from build123d import *

# Parameters (mm, degrees)
SKETCH1_W           = 150
SKETCH1_H           = 45
BOSS_EXTRUDE1_DEPTH = 60
SKETCH2_W           = 70
SKETCH2_H           = 30
CUT_EXTRUDE1_DEPTH  = 60
SKETCH8_W           = 25
SKETCH8_H           = 60
CUT_EXTRUDE5_DEPTH  = 30
SKETCH9_R           = 25
BOSS_EXTRUDE4_DEPTH = 35
SKETCH10_R          = 20
SKETCH10_R_2        = 15
CUT_EXTRUDE7_DEPTH  = 10
SKETCH10_5_R        = 15
SKETCH10_5_R_2      = 10
CUT_EXTRUDE8_DEPTH  = 70
SKETCH12_R          = 5
CUT_EXTRUDE9_DEPTH  = 70
FILLET1_R           = 10
SKETCH13_R          = 7
CUT_EXTRUDE10_DEPTH = 15
SKETCH14_R          = 5
CUT_EXTRUDE11_DEPTH = 15
FILLET2_R           = 5


with BuildPart() as part:
    # Sketch1 → Boss-Extrude1 (new body)
    with BuildSketch(Plane.XY):
        Rectangle(SKETCH1_W, SKETCH1_H)
    extrude(amount=BOSS_EXTRUDE1_DEPTH)

    # Sketch2 → Cut-Extrude1 (cut)
    with BuildSketch(Plane.XY.offset(60)):
        with Locations((0, -7.5)):
            Rectangle(SKETCH2_W, SKETCH2_H)
    extrude(amount=-CUT_EXTRUDE1_DEPTH, mode=Mode.SUBTRACT)

    # Sketch8 → Cut-Extrude5 (cut)
    with BuildSketch(Plane(origin=(0, 22.5, 0), x_dir=(1, 0, 0), z_dir=(0, 1, 0))):
        with Locations((-62.5, -30)):
            Rectangle(SKETCH8_W, SKETCH8_H)
        with Locations((62.5, -30)):
            Rectangle(SKETCH8_W, SKETCH8_H)
    extrude(amount=-CUT_EXTRUDE5_DEPTH, mode=Mode.SUBTRACT)

    # Sketch9 → Boss-Extrude4 (add)
    with BuildSketch(Plane(origin=(0, 22.5, 0), x_dir=(1, 0, 0), z_dir=(0, 1, 0))):
        with Locations(Location((0, -30, 0), (0, 0, 180))):
            Circle(SKETCH9_R)
    extrude(amount=BOSS_EXTRUDE4_DEPTH)

    # Sketch10 → Cut-Extrude7 (cut)
    with BuildSketch(Plane(origin=(0, 57.5, 0), x_dir=(1, 0, 0), z_dir=(0, 1, 0))):
        with Locations(Location((0, -30, 0), (0, 0, 270))):
            Circle(SKETCH10_R)
        with Locations(Location((0, -30, 0), (0, 0, 270))):
            Circle(SKETCH10_R_2, mode=Mode.SUBTRACT)
    extrude(amount=-CUT_EXTRUDE7_DEPTH, mode=Mode.SUBTRACT)

    # Sketch10_5 → Cut-Extrude8 (cut)
    # profile 1 of 2: a face of its own
    with BuildSketch(Plane(origin=(0, 57.5, 0), x_dir=(1, 0, 0), z_dir=(0, 1, 0))):
        with Locations(Location((0, -30, 0), (0, 0, 270))):
            Circle(SKETCH10_5_R)
        with Locations((0, -30)):
            Circle(SKETCH10_5_R_2, mode=Mode.SUBTRACT)
    # profile 2 of 2: a face of its own
    with BuildSketch(Plane(origin=(0, 57.5, 0), x_dir=(1, 0, 0), z_dir=(0, 1, 0))):
        with Locations((0, -30)):
            Circle(SKETCH10_5_R_2)
    extrude(amount=-CUT_EXTRUDE8_DEPTH, mode=Mode.SUBTRACT)

    # Sketch12 → Cut-Extrude9 (cut)
    with BuildSketch(Plane.XY.offset(60)):
        with Locations((0, 36.5)):
            Circle(SKETCH12_R)
    extrude(amount=-CUT_EXTRUDE9_DEPTH, mode=Mode.SUBTRACT)

    # Fillet1
    fillet1_edges = [part.edges().sort_by_distance(p)[0] for p in [
        (-75, -15, 0),
        (-75, -15, 60),
    ]]
    fillet(fillet1_edges, radius=FILLET1_R)

    # Sketch13 → Cut-Extrude10 (cut)
    with BuildSketch(Plane(origin=(0, -7.5, 0), x_dir=(1, 0, 0), z_dir=(0, 1, 0))):
        with Locations((75, -30)):
            Circle(SKETCH13_R)
    extrude(amount=-CUT_EXTRUDE10_DEPTH, mode=Mode.SUBTRACT)

    # Sketch14 → Cut-Extrude11 (cut)
    with BuildSketch(Plane(origin=(0, -7.5, 0), x_dir=(1, 0, 0), z_dir=(0, 1, 0))):
        with Locations(Location((-64.657240853, -15, 0), (0, 0, 180))):
            Circle(SKETCH14_R)
        with Locations(Location((-64.657240853, -45, 0), (0, 0, 180))):
            Circle(SKETCH14_R)
    extrude(amount=-CUT_EXTRUDE11_DEPTH, mode=Mode.SUBTRACT)

    # Fillet2
    fillet2_edges = [part.edges().sort_by_distance(p)[0] for p in [
        (-50, -7.5, 30),
        (-50, 22.5, 30),
        (50, -7.5, 30),
        (50, 22.5, 30),
    ]]
    fillet(fillet2_edges, radius=FILLET2_R)


solid = part.part
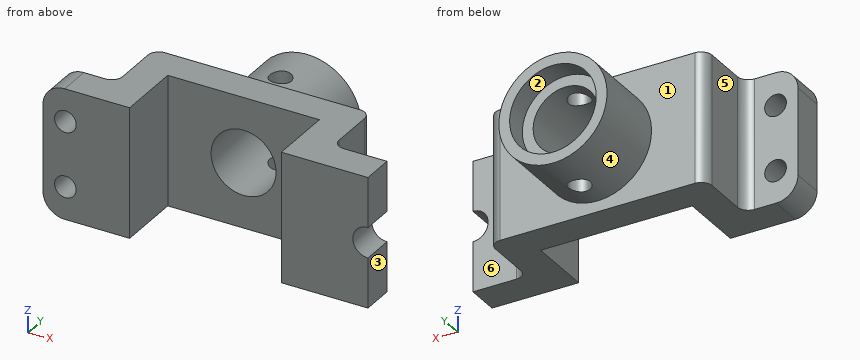
Can you work these out from the model? Positions are in its coordinate system, mm. Face numbers are marked on the shaded views. A direction names the side the tool comes from. Coordinates: 2 decimals unless noted, no trailing zeros. Loops run counter-clockwise (first coordinate to the right, second up) from the corner with the lowest first, then second, coordinate; pieces in that order, holes last. Notation, with made-up numbers: M 85.25,61 L 135.25,61 A20 cw 135.25,98 Z; hole C -36,-32.5 d3. An arc over 180 degrees is marked long. Answer as CSV lines item,"result". Start each with the question number.
1. For the marked faces 4, 5 and 6, which set-ups out of +Z, -Z, +X, -X, +Y, -Y let a thin tool reach every point of the face, with its end or its side?
2. If I drill on probe 1 along Y at (x, z) = (0, 7); probe 2 along X at (y, z) = (36, 10); probe 3 along X at (y, z) = (-1.5, 49), over which ranges is the centre line in solid material (lowest first)? Write a range as [from, to].
3. Suppose I cut it at A-A, the plane z = 30. List the corners of the cut face in (x, y) for me.
4. Thinking about a two-plate mould opening in X: for the marked faces 1, 2 and 3, which applies, +X half, -X half, draft (parallel to the pull), parting line (faces both ways), or undercut?
5. Suppose I cut it at D-D, the plane z = 11.5. Count the separate pieces of the cut face and the enclosed holes in it, plus the area to 3 significant figures.
6. Suppose I cut it at B-B, the plane y = -13.5. List the corners of the cut face in (x, z) for me.
7. For pin 1 Ø16 at (x, z) = (-63, 30.5) entering from +Y; pin 2 Ø20 at (x, z) = (9, 23) entering from +Y; pin 3 Ø3 at (x, z) = (-6.5, 19.5) entering from -Y; pin 4 Ø10 at (y, z) = (8, 23) entering from -X, each with a flat end and sliding along its axis, tell me the tip position at first contact or that it passes through.
8. Suppose I cut it at C-C, the plane x = 0. List the corners of the cut face in (y, z) for me.
Output:
1,face 4,"+Y"
1,face 5,"+Z, -Z, -X, +Y"
1,face 6,"+Z, -Z, +X, +Y"
2,probe 1,"y = [7.5, 31.5], [41.5, 57.5]"
2,probe 2,"x = [-15, -4.97], [4.97, 15]"
2,probe 3,"x = [-50, -35], [35, 50]"
3,outline,"M -75,-22.5 L -35,-22.5 L -35,7.5 L -15,7.5 L -15,47.5 L -20,47.5 L -20,57.5 L -25,57.5 L -25,22.5 L -45,22.5 A5 ccw -50,17.5 L -50,-2.5 A5 cw -55,-7.5 L -75,-7.5 Z; M 15,7.5 L 35,7.5 L 35,-22.5 L 68,-22.5 L 68,-7.5 L 55,-7.5 A5 cw 50,-2.5 L 50,17.5 A5 ccw 45,22.5 L 25,22.5 L 25,57.5 L 20,57.5 L 20,47.5 L 15,47.5 Z"
4,face 1,"draft"
4,face 2,"undercut"
4,face 3,"+X half"
5,separate pieces,"2"
5,enclosed holes,"1"
5,area,"3,990 mm^2"
6,outline,"M -75,10 A10 ccw -65,0 L -35,0 L -35,60 L -65,60 A10 ccw -75,50 Z; M 35,0 L 75,0 L 75,23 A7 cw 75,37 L 75,60 L 35,60 Z; hole C -64.66,15 d10; hole C -64.66,45 d10"
7,pin 1,"stops at y = -7.5"
7,pin 2,"stops at y = 57.5"
7,pin 3,"passes through"
7,pin 4,"stops at x = -50"
8,outline,"M 7.5,0 L 22.5,0 L 22.5,5 L 31.5,5 L 31.5,15 L 7.5,15 Z; M 7.5,45 L 31.5,45 L 31.5,55 L 22.5,55 L 22.5,60 L 7.5,60 Z; M 41.5,5 L 57.5,5 L 57.5,10 L 47.5,10 L 47.5,15 L 41.5,15 Z; M 41.5,45 L 47.5,45 L 47.5,50 L 57.5,50 L 57.5,55 L 41.5,55 Z"
